from build123d import *

# Parameters (mm, degrees)
F3_DEPTH  = 13
F4_T      = -1.2
F6_SIZE   = 1.8
F7_SIZE   = 1.2
F8_DEPTH  = 11.8
F10_DEPTH = 2


# Not quite as in the source:
# - a feature names something its author has since deleted; it is built from what else it names


with BuildPart() as f3:
    # F2 (on Top) → F3 (new body)
    with BuildSketch(Plane.XY):
        with BuildLine():
            ThreePointArc((-25, -21.3), (-23.9162950904, -23.9162950904), (-21.3, -25))
            Line((-21.3, -25), (21.3, -25))
            ThreePointArc((21.3, -25), (23.9162950904, -23.9162950904), (25, -21.3))
            Line((25, -21.3), (25, 21.3))
            ThreePointArc((25, 21.3), (23.9162950904, 23.9162950904), (21.3, 25))
            Line((21.3, 25), (-21.3, 25))
            ThreePointArc((-21.3, 25), (-23.9162950904, 23.9162950904), (-25, 21.3))
            Line((-25, 21.3), (-25, -21.3))
        make_face()
    extrude(amount=F3_DEPTH)

    # F4
    f4_openings = [f3.faces().sort_by_distance(p)[0] for p in [
        (0, 0, 13),
    ]]
    offset(amount=F4_T, openings=f4_openings)

    # F6
    f6_edges = [f3.edges().sort_by_distance(p)[0] for p in [
        (-23.916295, -23.916295, 0),
        (0, -25, 0),
        (23.916295, -23.916295, 0),
        (25, 0, 0),
        (23.916295, 23.916295, 0),
        (0, 25, 0),
        (-23.916295, 23.916295, 0),
        (-25, 0, 0),
    ]]
    chamfer(f6_edges, length=F6_SIZE)

    # F7
    f7_edges = [f3.edges().sort_by_distance(p)[0] for p in [
        (-23.067767, -23.067767, 1.2),
        (0, -23.8, 1.2),
        (23.067767, -23.067767, 1.2),
        (23.8, 0, 1.2),
        (23.067767, 23.067767, 1.2),
        (0, 23.8, 1.2),
        (-23.067767, 23.067767, 1.2),
        (-23.8, 0, 1.2),
    ]]
    chamfer(f7_edges, length=F7_SIZE)

    # F5 (on face) → F8 (join, through all)
    with BuildSketch(Plane.XY.offset(1.2)):
        with BuildLine():
            Line((-23.8, 18.8), (-21.3, 18.8))
            ThreePointArc((-21.3, 18.8), (-19.532233047, 19.532233047), (-18.8, 21.3))
            Line((-18.8, 21.3), (-18.8, 23.8))
            Line((-18.8, 23.8), (-21.3, 23.8))
            ThreePointArc((-21.3, 23.8), (-23.067766953, 23.067766953), (-23.8, 21.3))
            Line((-23.8, 21.3), (-23.8, 18.8))
        make_face()
        Polygon((-19.8734152256, 20.8364745084), (-21.3, 19.8), (-22.7265847744, 20.8364745084), (-22.1816778784, 22.5135254916), (-20.4183221216, 22.5135254916), align=None, mode=Mode.SUBTRACT)
        with BuildLine():
            Line((-21.3, -18.8), (-23.8, -18.8))
            Line((-23.8, -18.8), (-23.8, -21.3))
            ThreePointArc((-23.8, -21.3), (-23.067766953, -23.067766953), (-21.3, -23.8))
            Line((-21.3, -23.8), (-18.8, -23.8))
            Line((-18.8, -23.8), (-18.8, -21.3))
            ThreePointArc((-18.8, -21.3), (-19.532233047, -19.532233047), (-21.3, -18.8))
        make_face()
        Polygon((-22.7265847744, -21.7635254916), (-22.1816778784, -20.0864745084), (-20.4183221216, -20.0864745084), (-19.8734152256, -21.7635254916), (-21.3, -22.8), align=None, mode=Mode.SUBTRACT)
        with BuildLine():
            Line((21.3, 23.8), (18.8, 23.8))
            Line((18.8, 23.8), (18.8, 21.3))
            ThreePointArc((18.8, 21.3), (19.532233047, 19.532233047), (21.3, 18.8))
            Line((21.3, 18.8), (23.8, 18.8))
            Line((23.8, 18.8), (23.8, 21.3))
            ThreePointArc((23.8, 21.3), (23.067766953, 23.067766953), (21.3, 23.8))
        make_face()
        Polygon((19.8734152256, 20.8364745084), (20.4183221216, 22.5135254916), (22.1816778784, 22.5135254916), (22.7265847744, 20.8364745084), (21.3, 19.8), align=None, mode=Mode.SUBTRACT)
        with BuildLine():
            Line((18.8, -21.3), (18.8, -23.8))
            Line((18.8, -23.8), (21.3, -23.8))
            ThreePointArc((21.3, -23.8), (23.067766953, -23.067766953), (23.8, -21.3))
            Line((23.8, -21.3), (23.8, -18.8))
            Line((23.8, -18.8), (21.3, -18.8))
            ThreePointArc((21.3, -18.8), (19.532233047, -19.532233047), (18.8, -21.3))
        make_face()
        Polygon((19.8734152256, -21.7635254916), (20.4183221216, -20.0864745084), (22.1816778784, -20.0864745084), (22.7265847744, -21.7635254916), (21.3, -22.8), align=None, mode=Mode.SUBTRACT)
    extrude(amount=F8_DEPTH)

    # F9 (on face) → F10 (join)
    with BuildSketch(Plane.XY.offset(13)):
        with BuildLine():
            Line((-25, 21.3), (-25, -21.3))
            ThreePointArc((-25, -21.3), (-23.9162950904, -23.9162950904), (-21.3, -25))
            Line((-21.3, -25), (21.3, -25))
            ThreePointArc((21.3, -25), (23.9162950904, -23.9162950904), (25, -21.3))
            Line((25, -21.3), (25, 21.3))
            ThreePointArc((25, 21.3), (23.9162950904, 23.9162950904), (21.3, 25))
            Line((21.3, 25), (-21.3, 25))
            ThreePointArc((-21.3, 25), (-23.9162950904, 23.9162950904), (-25, 21.3))
        make_face()
        with BuildLine():
            ThreePointArc((-24.4, 21.3), (-23.4920310217, 23.4920310217), (-21.3, 24.4))
            Line((-21.3, 24.4), (21.3, 24.4))
            ThreePointArc((21.3, 24.4), (23.4920310217, 23.4920310217), (24.4, 21.3))
            Line((24.4, 21.3), (24.4, -21.3))
            ThreePointArc((24.4, -21.3), (23.4920310217, -23.4920310217), (21.3, -24.4))
            Line((21.3, -24.4), (-21.3, -24.4))
            ThreePointArc((-21.3, -24.4), (-23.4920310217, -23.4920310217), (-24.4, -21.3))
            Line((-24.4, -21.3), (-24.4, 21.3))
        make_face(mode=Mode.SUBTRACT)
    extrude(amount=F10_DEPTH)


solid = f3.part
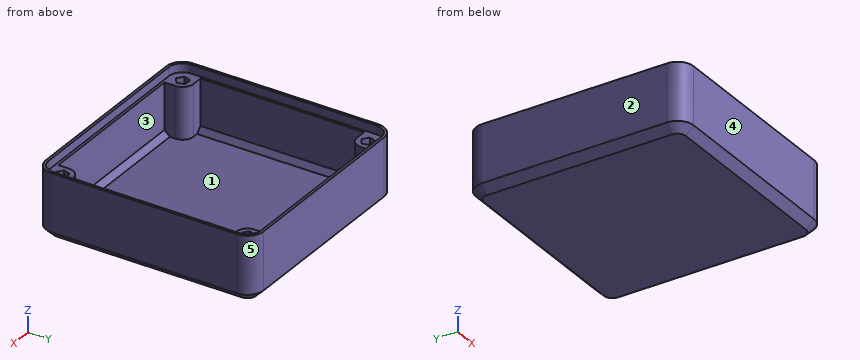
Check sheet for the modelled part. Datum: model origin and axes. Units: mm. Face numbers are marked on the shaded views. A direction names the side the tool comes from. Round coordinates to 2 decimals unless told otherwise and drop trailing zeros. Loops run counter-clockwise (first coordinate to the right, second up) from the corner with the lowest first, then second, coordinate; pieces in that order, holes last.
1. Sectioned sample at D-D on z = 4. Give the number of separate pieces and of enclosed holes in the cut face, and give its area (3 significant figures).
2. Sectioned sample at A-A on y = -8. Record the boundary of the cut face in (x, z), and give its area (3 significant figures).
3. Set-up check for the marked faces 1 and 2: record each of +Z, -Z, +X, -X, +Y, -Y from which the full face is reachable in a straight line by a thin tool's end or side.
4. Mould release check, pull along Y, two halves, no side actions. Record for the marked faces 3, 4 and 5: released by +Y, released by -Y, zero draft, split by the parting line, or undercut.
5. Scan lines: probe 1 along X at (y, z) = (-10.5, 3.5); probe 2 along Y at (x, z) = (-9, 14.25). Record each from-to range of solid material in increasing order.
6. Sectioned sample at B-B on z = 14.25. Record the boundary of the cut face in (x, y).
7. Gauge pin test, flat ends, axial feed: pin 1 Ø0.8 at (x, y) = (-21, -22) entering from +Z; pin 2 Ø24.5 at (x, y) = (7.5, 10.5) entering from +Z; pin 3 Ø2 at (x, z) = (-23, 4.5) entering from -Y. Record the tip position at first contact, or that the pin passes through.
Recorded:
1. separate pieces: 1
1. enclosed holes: 5
1. area: 296 mm2
2. outline: (-25, 1.8) - (-23.2, 0) - (23.2, 0) - (25, 1.8) - (25, 15) - (24.4, 15) - (24.4, 13) - (23.8, 13) - (23.8, 2.4) - (22.6, 1.2) - (-22.6, 1.2) - (-23.8, 2.4) - (-23.8, 13) - (-24.4, 13) - (-24.4, 15) - (-25, 15) - close
2. area: 88.9 mm2
3. face 1: +Z
3. face 2: +Z, -Z, -X, +Y, -Y
4. face 3: undercut
4. face 4: released by -Y
4. face 5: released by +Y
5. probe 1: x = -25 to -23.8, 23.8 to 25
5. probe 2: y = -25 to -24.4, 24.4 to 25
6. outline: (-25, -21.3) arc R3.7 ccw to (-21.3, -25) - (21.3, -25) arc R3.7 ccw to (25, -21.3) - (25, 21.3) arc R3.7 ccw to (21.3, 25) - (-21.3, 25) arc R3.7 ccw to (-25, 21.3) - close; hole (-24.4, -21.3) arc R3.1 ccw to (-21.3, -24.4) - (21.3, -24.4) arc R3.1 ccw to (24.4, -21.3) - (24.4, 21.3) arc R3.1 ccw to (21.3, 24.4) - (-21.3, 24.4) arc R3.1 ccw to (-24.4, 21.3) - close
7. pin 1: stops at z = 1.2
7. pin 2: stops at z = 1.35
7. pin 3: stops at y = -24.93
